Source: three-view drawing plus pictorial views. Frame: mm from the lowest corner of the part. A direction names the side the tool comes from. Give positions to 0.01 mm unless a question says otherwise; leave off trailing zeros. Loops run counter-clockwise (first coordinate to the right, second up) from the corner with the lowest first, then second, coordinate; pieces in that order, holes last. Notation, with made-up numbers: M 89,62 L 124,62 A25 cw 124,98 Z; hole C 30.25,58 d6. An arc over 180 degrees is marked long. Answer as a JSON object with one key per item and string values. Group by question number.
1) Access query for the marked faces 1, 2 and 3. Directions: +Z, -Z, +X, -X, +Y, -Y. A direction counts if a zero-diameter tool reaches every point of the face in a straight line with its end or side. Return the directions, or none.
2) Section query B-B on x = 10. Return loops of the section in (y, z), plus the area to 3 significant figures.
3) Section query C-C on z = 0.75. Return loops of the section in (x, y).
4) Section query D-D on y = 19. Return loops of the section in (x, z), plus the area to 3 significant figures.
5) First-contact query: P1, Ø6, axis at y = 52, z = 2, coming from the -X side; P2, Ø2.5, axis at x = 11.5, z = 5.5, coming from the +Y side; P3, Ø5, axis at y = 25.5, z = 3, coming from the +X side; P4, Ø6, axis at x = 9.5, y = 34.5, coming from the +Z side. Flat tips, straight axial feed; report the tip coordinate or a pass-through.
6) Ray query, L1, parallel to Z at x = 9.5, y = 1.4; L2, parallel to Y at x = 2.25, z = 6.5; L3, parallel to X at y = 53, z = 3.25. Return the intervals inside material, ascending.
7) Section query A-A on z = 5. Return loops of the section in (x, y).
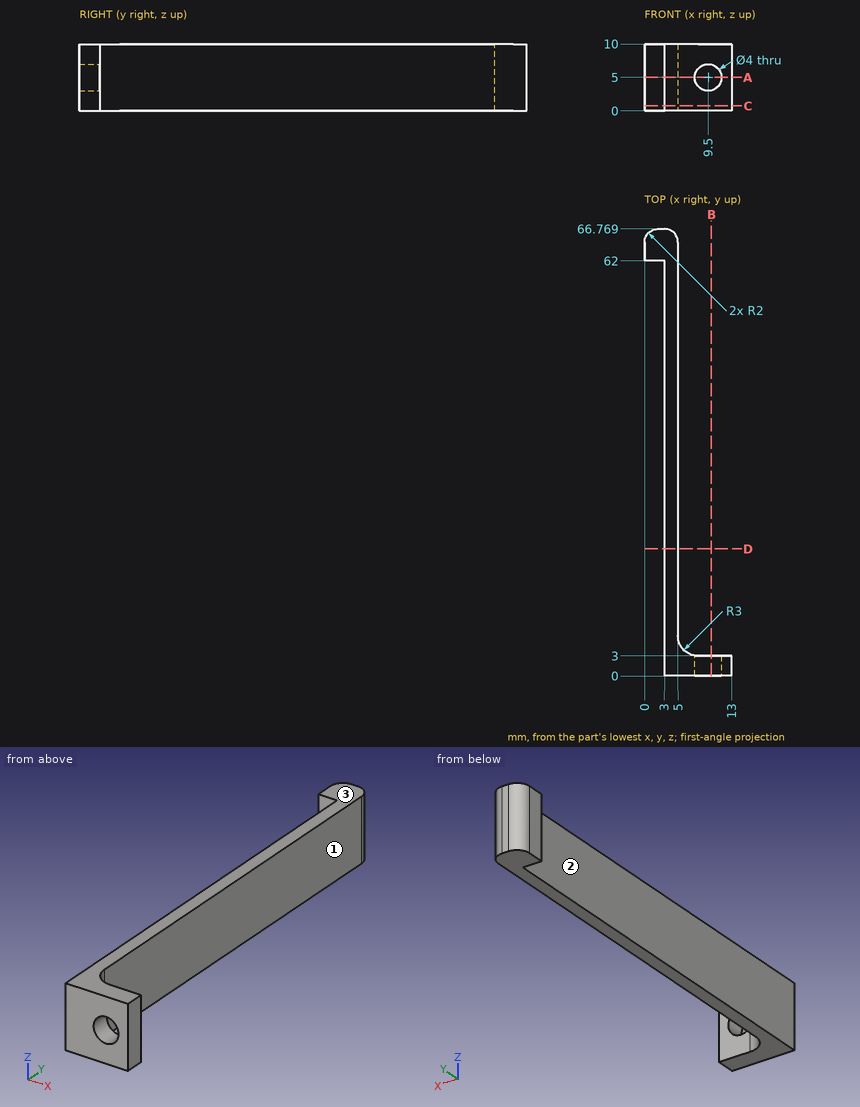
Output:
{
 "1": {"face 1": "+Z, -Z, +X, +Y", "face 2": "+Z, -Z, -X, -Y", "face 3": "+Z, +X, -X, +Y, -Y"},
 "2": {"outline": "M 0,0 L 3,0 L 3,3.06 L 0,3.06 Z; M 0,6.94 L 3,6.94 L 3,10 L 0,10 Z", "area": "18.4 mm^2"},
 "3": {"outline": "M 0,62 L 3,62 L 3,0 L 13,0 L 13,3 L 8,3 A3 cw 5,6 L 5,64.77 A2 ccw 3,66.77 L 2,66.77 A2 ccw 0,64.77 Z"},
 "4": {"outline": "M 3,0 L 5,0 L 5,10 L 3,10 Z", "area": "20.0 mm^2"},
 "5": {"P1": "stops at x = 3", "P2": "stops at y = 3", "P3": "stops at x = 5", "P4": "passes through"},
 "6": {"L1": "z = 0 to 3, 7 to 10", "L2": "y = 62 to 66.77", "L3": "x = 3 to 5"},
 "7": {"outline": "M 0,62 L 3,62 L 3,0 L 7.5,0 L 7.5,3.04 A3 cw 5,6 L 5,64.77 A2 ccw 3,66.77 L 2,66.77 A2 ccw 0,64.77 Z; M 11.5,0 L 13,0 L 13,3 L 11.5,3 Z"}
}
